```python
from build123d import *

# Parameters (mm, degrees)
F1_DEPTH = 3
F2_R     = 3
F3_DEPTH = 25
F6_DEPTH = 25
F8_DEPTH = 3


with BuildPart() as f1:
    # F0 (on Front) → F1 (new body)
    with BuildSketch(Plane.XZ):
        with BuildLine():
            ThreePointArc((5.9371710435, 0), (10.73463176, 4.595495259), (12.5, 11))
            ThreePointArc((12.5, 11), (0, 23.5), (-12.5, 11))
            ThreePointArc((-12.5, 11), (-10.73463176, 4.595495259), (-5.9371710435, 0))
            Line((-5.9371710435, 0), (5.9371710435, 0))
        make_face()
        with BuildLine():
            ThreePointArc((-5.9371710435, 0), (-10.73463176, 4.595495259), (-12.5, 11))
            Line((-12.5, 11), (-12.5, 0))
            Line((-12.5, 0), (-5.9371710435, 0))
        make_face()
    extrude(amount=F1_DEPTH)

    # F2 (on face) → F3 (cut)
    with BuildSketch(Plane.XZ.offset(3)):
        with Locations((0, 11)):
            Circle(F2_R)
    extrude(amount=-F3_DEPTH, mode=Mode.SUBTRACT)

    # F4: F1 across face


with BuildPart() as f1_1:
    add(f1.part)
    add(f1.part.mirror(Plane(origin=(-3.2814144782, -1.5, 0), x_dir=(1, 0, 0), z_dir=(0, 0, -1))))

    # F5 (on face) → F6 (cut)
    with BuildSketch(Plane.XZ.offset(3)):
        with BuildLine():
            ThreePointArc((-7.80859375, -12.7395009766), (-8, -11), (-7.80859375, -9.2604990234))
            ThreePointArc((-7.80859375, -9.2604990234), (-9.75, -11), (-7.80859375, -12.7395009766))
        make_face()
        with BuildLine():
            ThreePointArc((-6.25, -11), (-6.6966464529, -9.8321945662), (-7.80859375, -9.2604990234))
            ThreePointArc((-7.80859375, -9.2604990234), (-8, -11), (-7.80859375, -12.7395009766))
            ThreePointArc((-7.80859375, -12.7395009766), (-6.6966464529, -12.1678054338), (-6.25, -11))
        make_face()
        with BuildLine():
            ThreePointArc((7.80859375, -9.2604990234), (7.9520044643, -10.125), (8, -11))
            ThreePointArc((8, -11), (7.9520044643, -11.875), (7.80859375, -12.7395009766))
            ThreePointArc((7.80859375, -12.7395009766), (9.1678054338, -12.3033535471), (9.75, -11))
            ThreePointArc((9.75, -11), (9.1678054338, -9.6966464529), (7.80859375, -9.2604990234))
        make_face()
        with BuildLine():
            ThreePointArc((7.80859375, -12.7395009766), (7.9520044643, -11.875), (8, -11))
            ThreePointArc((8, -11), (7.9520044643, -10.125), (7.80859375, -9.2604990234))
            ThreePointArc((7.80859375, -9.2604990234), (6.25, -11), (7.80859375, -12.7395009766))
        make_face()
    extrude(amount=-F6_DEPTH, mode=Mode.SUBTRACT)

    # F7 (on face) → F8 (join)
    with BuildSketch(Plane.XZ.offset(3)):
        with BuildLine():
            Line((12.5, -11), (12.5, 11))
            ThreePointArc((12.5, 11), (10.73463176, 4.595495259), (5.9371710435, 0))
            ThreePointArc((5.9371710435, 0), (10.73463176, -4.595495259), (12.5, -11))
        make_face()
    extrude(amount=-F8_DEPTH)


solid = f1_1.part
```
Build history of the part. All positions in model axes, mm. Give positions to 0.01 mm unless a question says otherwise; leave off trailing zeros. Loops run counter-clockwise (first coordinate to the right, second up) from the corner with the lowest first, then second, coordinate; pieces in that order, holes last.
1) Band-saw the part on A-A on y = -2. List the corners of the cut face in (x, z).
Values follow:
outline: (-12.5, -11) arc R12.5 ccw to (12.5, -11) - (12.5, 11) arc R12.5 ccw to (-12.5, 11) - close; hole circle Ø3.5 at (-8, -11); hole circle Ø6 at (0, -11); hole circle Ø6 at (0, 11); hole circle Ø3.5 at (8, -11)
2) Band-saw the part on D-D on z = 12. List the corners of the cut face in (x, y), then the cut area to 3 significant figures.
Values follow:
outline: (-12.46, -3) - (-2.83, -3) - (-2.83, 0) - (-12.46, 0) - close; (2.83, -3) - (12.46, -3) - (12.46, 0) - (2.83, 0) - close
area: 57.8 mm2
3) Band-saw the part on B-B on x = 0. List the corners of the cut face in (y, z).
Values follow:
outline: (-3, -23.5) - (0, -23.5) - (0, -14) - (-3, -14) - close; (-3, -8) - (0, -8) - (0, 8) - (-3, 8) - close; (-3, 14) - (0, 14) - (0, 23.5) - (-3, 23.5) - close
4) Two-plate mould, pull along X, no slides. Class faces 1 (the face through (0, 0, 0)), 2 (the face through (0.275, -1.479, 23.497)), 3 (the face through (-0.65, -1.52, -8.07)): released by +X, released by -X, zero draft, split by the parting line, or undercut.
Values follow:
face 1: zero draft
face 2: split by the parting line
face 3: undercut
5) Probe line 1 along Z through (x, y) = (0, -0.95); line 2 along Z through (x, y) = (2.5, -2.35); line 3 along X through (y, z) = (-2.2, 12.5). List the from-to ranges inside material, lowest first.
Values follow:
line 1: z = -23.5 to -14, -8 to 8, 14 to 23.5
line 2: z = -23.25 to -12.66, -9.34 to 9.34, 12.66 to 23.25
line 3: x = -12.41 to -2.6, 2.6 to 12.41
6) Band-saw the part on C-C on z = -10.5. List the corners of the cut face in (x, y).
Values follow:
outline: (-12.5, -3) - (-9.68, -3) - (-9.68, 0) - (-12.5, 0) - close; (-6.32, -3) - (-2.96, -3) - (-2.96, 0) - (-6.32, 0) - close; (2.96, -3) - (6.32, -3) - (6.32, 0) - (2.96, 0) - close; (9.68, -3) - (12.5, -3) - (12.5, 0) - (9.68, 0) - close
7) Drop flat-ended pins along their axis: P1, Ø1.5, axis at x = -8.5, y = -1, coming from the +Z side; P2, Ø5, axis at x = 0, z = -11, coming from the +Y side. Give the stop position or say it passes through.
Values follow:
P1: stops at z = 20.81
P2: passes through
